The listing builds one solid part. Answer for the finished solid, in the listing's coordinates (mm). Round coordinates to 2 decimals unless told otherwise and drop trailing zeros. Answer in a Markdown table with one row per item. Add a question column.
```python
from build123d import *

# Parameters (mm, degrees)
SKETCH1_R           = 70
BOSS_EXTRUDE1_DEPTH = 50
SKETCH3_R           = 65
CUT_EXTRUDE1_DEPTH  = 45
CUT_EXTRUDE2_DEPTH  = 82.5
FILLET2_R           = 7
SKETCH5_R           = 50
BOSS_EXTRUDE2_DEPTH = 2


with BuildPart() as part:
    # Sketch1 → Boss-Extrude1 (new body)
    with BuildSketch(Plane(origin=(0, 0, 0), x_dir=(0, 0, -1), z_dir=(1, 0, 0))):
        Circle(SKETCH1_R)
    extrude(amount=BOSS_EXTRUDE1_DEPTH)

    # Sketch3 → Cut-Extrude1 (cut)
    with BuildSketch(Plane(origin=(50, 0, 0), x_dir=(0, 0, -1), z_dir=(1, 0, 0))):
        Circle(SKETCH3_R)
    extrude(amount=-CUT_EXTRUDE1_DEPTH, mode=Mode.SUBTRACT)

    # Sketch4 → Cut-Extrude2 (cut, symmetric)
    with BuildSketch(Plane(origin=(0, 0, 0), x_dir=(1, 0, 0), z_dir=(0, 1, 0))):
        with BuildLine():
            Line((50, -70), (50, 70))
            Line((50, 70), (10, 70))
            add(Edge.make_bspline(
                [(10, 70), (8.736205307, 29.113153139), (29.458127412, -5.568528558), (46.811482452, -55.943406632), (50, -70)],
                knots=[0, 0, 0, 0, 0.596241342, 1, 1, 1, 1], degree=3))
        make_face()
    extrude(amount=CUT_EXTRUDE2_DEPTH, both=True, mode=Mode.SUBTRACT)

    # Fillet2
    fillet2_edges = [part.edges().sort_by_distance(p)[0] for p in [
        (0, 0, 70),
    ]]
    fillet(fillet2_edges, radius=FILLET2_R)

    # Sketch5 → Boss-Extrude2 (add)
    with BuildSketch(Plane.ZY):
        Circle(SKETCH5_R)
    extrude(amount=BOSS_EXTRUDE2_DEPTH)


solid = part.part
```
1. Straight lines are drawn through the part: line 1 along Y through (x, z) = (17.5, 0); line 2 along X through (y, z) = (6, -38); line 3 along Z through (x, y) = (43, 1). For each, find the intervals that lie inside material, in ascending order.
2. The mould has two halves that part along Y. Classify faces 1 (the flat face through (-2, 1, -1)), 2 (the cylindrical face through (23.421, 3.078, 69.932)), 3 (the flat face through (5, 1, 1)), 4 (the cylindrical face through (22.33, 2.858, 64.937)): released by +Y, released by -Y, zero draft, split by the parting line, or undercut.
3. Each of these flat-tipped pins is pushed along its axis until it touches: pin 1 (3 mm diameter, centred on x = 17, y = 33.5, fed in from -Z); pin 2 (10 mm diameter, centred on y = 3, z = 36.5, fed in from +X); pin 3 (1 mm diameter, centred on x = 6, z = -39.5, fed in from +Y). Where does it stop, or does it pass through?
Report:
| question | item | result |
|---|---|---|
| 1 | line 1 | y = -70 to -65, 65 to 70 |
| 1 | line 2 | x = -2 to 5 |
| 1 | line 3 | z = 64.99 to 69.99 |
| 2 | face 1 | zero draft |
| 2 | face 2 | split by the parting line |
| 2 | face 3 | undercut |
| 2 | face 4 | undercut |
| 3 | pin 1 | stops at z = 54.77 |
| 3 | pin 2 | stops at x = 5 |
| 3 | pin 3 | stops at y = 58.05 |
